```python
from build123d import *

# Parameters (mm, degrees)
SKETCH1_W           = 19
SKETCH1_H           = 50.8
SKETCH1_R           = 3.375
BOSS_EXTRUDE1_DEPTH = 14
BOSS_EXTRUDE2_DEPTH = 5
SKETCH2_R           = 12.7
CUT_EXTRUDE1_DEPTH  = 57.014640943


with BuildPart() as part:
    # Sketch1 → Boss-Extrude1 (new body)
    with BuildSketch(Plane(origin=(0, 0, 0), x_dir=(1, 0, 0), z_dir=(0, 1, 0))):
        with Locations((9.5, 25.4)):
            Rectangle(SKETCH1_W, SKETCH1_H)
        with Locations(Location((9.5, 44.45, 0), (0, 0, 270))):
            Circle(SKETCH1_R, mode=Mode.SUBTRACT)
        with Locations(Location((9.5, 6.35, 0), (0, 0, 270))):
            Circle(SKETCH1_R, mode=Mode.SUBTRACT)
    extrude(amount=-BOSS_EXTRUDE1_DEPTH)

    # Sketch1_3 → Boss-Extrude2 (add)
    with BuildSketch(Plane(origin=(0, 0, 0), x_dir=(1, 0, 0), z_dir=(0, 1, 0))):
        with BuildLine():
            Line((0, 38.1), (0, 12.7))
            ThreePointArc((0, 12.7), (9.5, 14.679128857), (19, 12.7))
            Line((19, 12.7), (19, 38.1))
            ThreePointArc((19, 38.1), (9.5, 36.120871143), (0, 38.1))
        make_face()
    extrude(amount=BOSS_EXTRUDE2_DEPTH)

    # Sketch2 → Cut-Extrude1 (cut, through all)
    with BuildSketch(Plane(origin=(19, 0, 0), x_dir=(0, 0, -1), z_dir=(1, 0, 0))):
        with Locations((25.4, -14)):
            Circle(SKETCH2_R)
    extrude(amount=-CUT_EXTRUDE1_DEPTH, mode=Mode.SUBTRACT)


solid = part.part
```
Design review of the part built by this model. Coordinates are the model's own, in mm. A direction names the side the tool comes from. Give positions to 0.01 mm unless a question says otherwise; leave off trailing zeros. Write each loop counter-clockwise with the first axis right and the second up, starting at its lowest first coordinate (ties: lowest second). Pieces come first, ordered by that corner, then holes. Notation, with made-up numbers: (32.25, 8.25) -> (88.25, 8.25) arc R27 ccw to (88.25, 38.25) -> close; hole circle Ø1 at (-30.5, 79.25). An arc over 180 degrees is marked (long way). Answer in a Markdown table with one row per item.
(1) Clearance check with flat-ended pins moving along their axes: pin 1 (3 mm diameter, centred on x = 4, y = 3, fed in from +Z); pin 2 (2 mm diameter, centred on x = 13.5, z = -36, fed in from -Y); pin 3 (7.5 mm diameter, centred on x = 8, z = -46.5, fed in from +Y). State where each tip first meets the part, or that it passes through.
Results:
| item | result |
|---|---|
| pin 1 | z = -13.63 |
| pin 2 | y = -8.83 |
| pin 3 | y = 0 |
(2) Consider section C-C (y = -5.75). State the section outline as (x, z) points (3 decimals).
Results:
| item | result |
|---|---|
| outline | (0, -50.8) -> (19, -50.8) -> (19, -35.055) -> (0, -35.055) -> close; (0, -15.745) -> (19, -15.745) -> (19, 0) -> (0, 0) -> close; hole circle Ø6.75 at (9.5, -44.45); hole circle Ø6.75 at (9.5, -6.35) |
(3) To check wall thickness, follow probe 1 along Z at (x, y) = (7.5, -3); probe 2 along Z at (x, y) = (8, -3); probe 3 along Z at (x, y) = (16, -11.25). State the ranges of each line that lie inside material, in increasing order.
Results:
| item | result |
|---|---|
| probe 1 | -50.8 to -47.17, -41.73 to -31.75, -19.05 to -9.07, -3.63 to 0 |
| probe 2 | -50.8 to -47.47, -41.43 to -31.75, -19.05 to -9.37, -3.33 to 0 |
| probe 3 | -50.8 to -37.8, -13 to 0 |
(4) Mouldability with a two-part tool opening along X and no side actions: class faces 4 (the flat face through (7, -14, -47)), 5 (the flat face through (0, 0, -25)), 6 (the cylindrical face through (11.78, -6.9, -8.84)) as +X half, -X half, draft (parallel to the pull), parting line (faces both ways), or undercut.
Results:
| item | result |
|---|---|
| face 4 | draft |
| face 5 | -X half |
| face 6 | undercut |
(5) Consider section D-D (z = -37). State the section outline as (x, y) points, then the cut area to 3 significant figures.
Results:
| item | result |
|---|---|
| outline | (0, -8.83) -> (19, -8.83) -> (19, 5) -> (15.91, 5) -> (15.91, 0) -> (3.09, 0) -> (3.09, 5) -> (0, 5) -> close |
| area | 199 mm2 |
(6) Consider section B-B (x = 9.5). State the section outline as (y, z) points (3 decimals), then the cut area to 3 significant figures.
Results:
| item | result |
|---|---|
| outline | (-14, -50.8) -> (0, -50.8) -> (0, -47.825) -> (-14, -47.825) -> close; (-14, -41.075) -> (0, -41.075) -> (0, -36.121) -> (5, -36.121) -> (5, -14.679) -> (0, -14.679) -> (0, -9.725) -> (-14, -9.725) -> (-14, -12.7) arc R12.7 cw to (-14, -38.1) -> close; (-14, -2.975) -> (0, -2.975) -> (0, 0) -> (-14, 0) -> close |
| area | 376 mm2 |
(7) For faces 1 (the cylindrical face through (9.64, 2.46, -36.12)), 2 (the flat face through (9, 5, -26)), 3 (the cylindrical face through (9.36, 2.46, -14.68)), list the 3-axis set-ups (+Z, -Z, +X, -X, +Y, -Y) from which the entire face can be reached by the end or side of a thin tool; tool diameter is ignored.
Results:
| item | result |
|---|---|
| face 1 | -Z, +Y |
| face 2 | +Z, -Z, +X, -X, +Y |
| face 3 | +Z, +Y |
(8) Consider section A-A (z = -6.35). State the section outline as (x, y) points (3 decimals), then the cut area to 4 significant figures.
Results:
| item | result |
|---|---|
| outline | (0, -14) -> (6.125, -14) -> (6.125, 0) -> (0, 0) -> close; (12.875, -14) -> (19, -14) -> (19, 0) -> (12.875, 0) -> close |
| area | 171.5 mm2 |
